Check sheet for the drawn part. Datum: minimum x, y, z corner. Units: mm. Give positions to 0.01 mm unless a question says otherwise; leave off trailing zeros. Loops run counter-clockwise (first coordinate to the right, second up) from the corner with the lowest first, then second, coordinate; pieces in that order, holes last. Notation, with made-up numbers: (-35, 17.5) - (-24, 17.5) arc R14 ccw to (-24, 41.5) - close; hole circle Ø6 at (-24, -20). An arc over 180 degrees is marked (long way). Use one line per item in the form item = value.
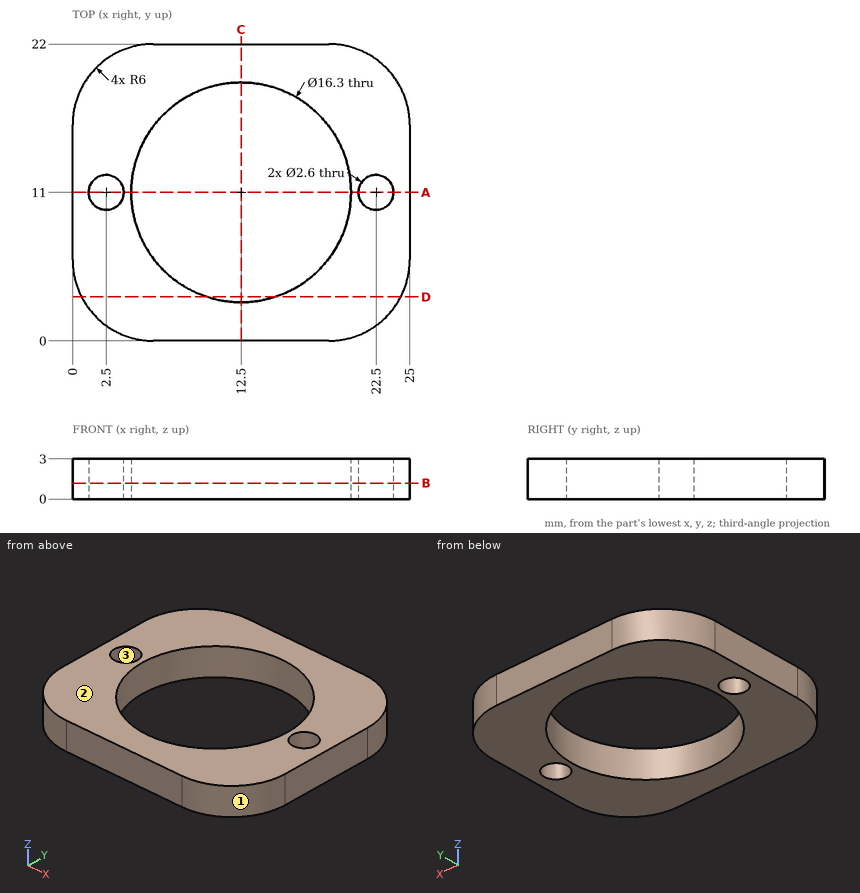
Item 1: Mould release check, pull along X, two halves, no side actions. Record for the marked faces 1, 2 and 3: released by +X, released by -X, zero draft, split by the parting line, or undercut.
Answer block:
face_1 = released by +X
face_2 = zero draft
face_3 = undercut
Item 2: Thickness scan on L1, parallel to Y at x = 12.5, z = 1; L2, parallel to X at y = 15, z = 0.65; L3, parallel to Y at x = 5.5, z = 1.55. Record the ranges inside material, lowest first.
Answer block:
L1 = 0 to 2.85, 19.15 to 22
L2 = 0 to 5.4, 19.6 to 25
L3 = 0.02 to 6.83, 15.17 to 21.98
Item 3: Gauge pin test, flat ends, axial feed: P1, Ø2.5, axis at x = 2.5, y = 11, coming from the -Z side; P2, Ø1.5, axis at x = 22.5, z = 0.5, coming from the -Y side. Record the tip position at first contact, or that the pin passes through.
Answer block:
P1 = through
P2 = 0.67
Item 4: Section check B-B on z = 1.2. Record the boundary of the cut face in (x, y), then the cut area to 3 significant figures.
Answer block:
outline = (0, 6) arc R6 ccw to (6, 0) - (19, 0) arc R6 ccw to (25, 6) - (25, 16) arc R6 ccw to (19, 22) - (6, 22) arc R6 ccw to (0, 16) - close; hole circle Ø2.6 at (2.5, 11); hole circle Ø16.3 at (12.5, 11); hole circle Ø2.6 at (22.5, 11)
area = 300 mm2
Item 5: Section check C-C on x = 12.5. Record the boundary of the cut face in (y, z), then the cut area to 3 significant figures.
Answer block:
outline = (0, 0) - (2.85, 0) - (2.85, 3) - (0, 3) - close; (19.15, 0) - (22, 0) - (22, 3) - (19.15, 3) - close
area = 17.1 mm2
Item 6: Section check A-A on y = 11. Record the boundary of the cut face in (x, z).
Answer block:
outline = (0, 0) - (1.2, 0) - (1.2, 3) - (0, 3) - close; (3.8, 0) - (4.35, 0) - (4.35, 3) - (3.8, 3) - close; (20.65, 0) - (21.2, 0) - (21.2, 3) - (20.65, 3) - close; (23.8, 0) - (25, 0) - (25, 3) - (23.8, 3) - close
Item 7: Section check D-D on y = 3.25. Record the boundary of the cut face in (x, z), then the cut area to 3 significant figures.
Answer block:
outline = (0.67, 0) - (9.98, 0) - (9.98, 3) - (0.67, 3) - close; (15.02, 0) - (24.33, 0) - (24.33, 3) - (15.02, 3) - close
area = 55.9 mm2
